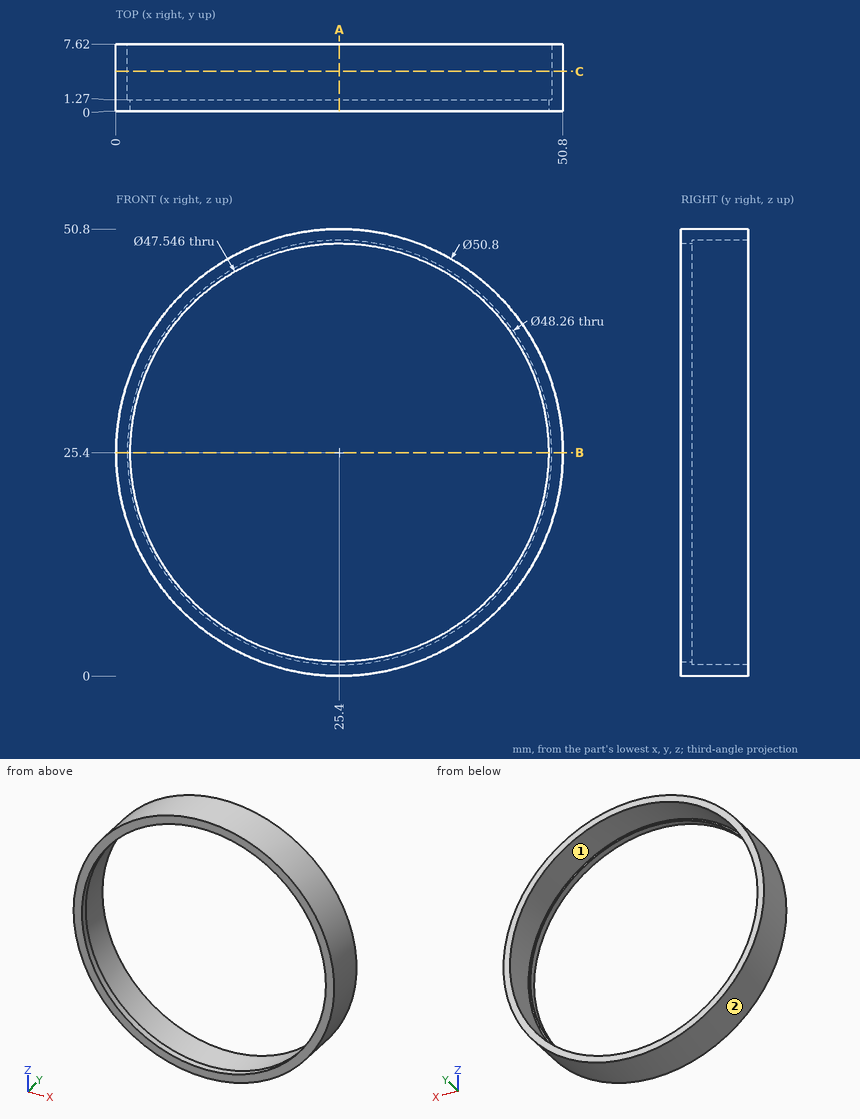
Print and shaded views of the part. All mm, measured from the part's lowest x, y and z. Round coordinates to 2 decimals unless told otherwise and drop trailing zeros. Write each loop counter-clockwise with the first axis right and the second up, starting at its lowest first coordinate (ties: lowest second). Pieces come first, ordered by that corner, then holes. Notation, with made-up numbers: (77.5, 30.25) - (112.5, 30.25) arc R25 cw to (112.5, 68.25) - close; hole circle Ø5 at (6, -7). An arc over 180 degrees is marked (long way). Use CSV: the item, a comma, the result in double quotes. Start each with the question number.
Item 1: Band-saw the part on A-A (x = 25.4). Write the cut outline in (y, z).
Item 2: Band-saw the part on B-B (z = 25.4). Write the cut outline in (x, y).
Item 3: Two-plate mould, pull along X, no slides. Class the marked faces 1 and 2: released by +X, released by -X, zero draft, split by the parting line, or undercut.
Item 4: Drill centre lines: L1, parallel to Z at x = 25.4, y = 1.05; L2, parallel to Z at x = 25.4, y = 3.75. Where is each one in solid material? Low to high. Write a range as [from, to].
Item 5: Pin check, flat tips, straight feed: P1, Ø4, axis at x = 17.5, y = 6, coming from the +Z side (1 decimal); P2, Ø2, axis at y = 1, z = 42, coming from the -X side (1 decimal); P3, Ø1, axis at y = 1.5, z = 14.5, coming from the +X side. Stop position of each tip, or through.
Item 6: Band-saw the part on C-C (y = 4.5). Write the cut outline in (x, z).
Checked values:
1,outline,"(0, 0) - (7.62, 0) - (7.62, 1.27) - (1.27, 1.27) - (1.27, 1.63) - (0, 1.63) - close; (0, 49.17) - (1.27, 49.17) - (1.27, 49.53) - (7.62, 49.53) - (7.62, 50.8) - (0, 50.8) - close"
2,outline,"(0, 0) - (1.63, 0) - (1.63, 1.27) - (1.27, 1.27) - (1.27, 7.62) - (0, 7.62) - close; (49.17, 0) - (50.8, 0) - (50.8, 7.62) - (49.53, 7.62) - (49.53, 1.27) - (49.17, 1.27) - close"
3,face 1,"undercut"
3,face 2,"split by the parting line"
4,L1,"z = [0, 1.63], [49.17, 50.8]"
4,L2,"z = [0, 1.27], [49.53, 50.8]"
5,P1,"stops at z = 50.1"
5,P2,"stops at x = 5.4"
5,P3,"stops at x = 48.57"
6,outline,"circle Ø50.8 at (25.4, 25.4); hole circle Ø48.26 at (25.4, 25.4)"
